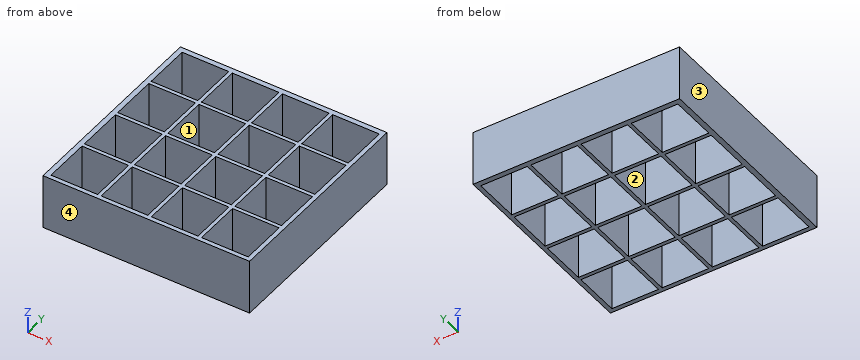
```python
from build123d import *

# Parameters (mm, degrees)
F0_W     = 1463.675
F0_H     = 1463.675
F0_W_2   = 330.2
F0_H_2   = 330.2
F1_DEPTH = 390.525
F2_SCALE = 0.05


with BuildPart() as f1:
    # F0 (on Top) → F1 (new body)
    with BuildSketch(Plane.XY):
        Rectangle(F0_W, F0_H)
        with Locations((-530.225, -536.575)):
            Rectangle(F0_W_2, F0_H_2, mode=Mode.SUBTRACT)
        with Locations((-174.625, -536.575)):
            Rectangle(F0_W_2, F0_H_2, mode=Mode.SUBTRACT)
        with Locations((-530.225, -180.975)):
            Rectangle(F0_W_2, F0_H_2, mode=Mode.SUBTRACT)
        with Locations((-174.625, -180.975)):
            Rectangle(F0_W_2, F0_H_2, mode=Mode.SUBTRACT)
        with Locations((180.975, -536.575)):
            Rectangle(F0_W_2, F0_H_2, mode=Mode.SUBTRACT)
        with Locations((536.575, -536.575)):
            Rectangle(F0_W_2, F0_H_2, mode=Mode.SUBTRACT)
        with Locations((180.975, -180.975)):
            Rectangle(F0_W_2, F0_H_2, mode=Mode.SUBTRACT)
        with Locations((536.575, -180.975)):
            Rectangle(F0_W_2, F0_H_2, mode=Mode.SUBTRACT)
        with Locations((-530.225, 174.625)):
            Rectangle(F0_W_2, F0_H_2, mode=Mode.SUBTRACT)
        with Locations((-174.625, 174.625)):
            Rectangle(F0_W_2, F0_H_2, mode=Mode.SUBTRACT)
        with Locations((-530.225, 530.225)):
            Rectangle(F0_W_2, F0_H_2, mode=Mode.SUBTRACT)
        with Locations((-174.625, 530.225)):
            Rectangle(F0_W_2, F0_H_2, mode=Mode.SUBTRACT)
        with Locations((180.975, 174.625)):
            Rectangle(F0_W_2, F0_H_2, mode=Mode.SUBTRACT)
        with Locations((536.575, 174.625)):
            Rectangle(F0_W_2, F0_H_2, mode=Mode.SUBTRACT)
        with Locations((180.975, 530.225)):
            Rectangle(F0_W_2, F0_H_2, mode=Mode.SUBTRACT)
        with Locations((536.575, 530.225)):
            Rectangle(F0_W_2, F0_H_2, mode=Mode.SUBTRACT)
    extrude(amount=F1_DEPTH)


with BuildPart() as f1_1:
    # F2: moved
    add(f1.part.scale(F2_SCALE))


solid = f1_1.part
```
Input: part model. Units: mm. Frame: model coordinates. Face numbers are marked on the shaded views. Coordinates: 2 decimals unless noted, no trailing zeros. Write each loop counter-clockwise with the first axis right and the second up, starting at its lowest first coordinate (ties: lowest second). Pieces come first, ordered by that corner, then holes. Notation, with made-up numbers: M 71,76 L 110,76 A20 cw 110,89 Z; hole C 85,-22.5 d2. An arc over 180 degrees is marked long. Use one line per item in the form item = value.
Q1. Section C-C (z = 1.5). Count the separate pieces of the cut face and the enclosed holes in it, plus the area to 3 significant figures.
Answer below:
separate_pieces = 1
enclosed_holes = 16
area = 995 mm²
Q2. Material intervals for probe 1 along X at (y, z) = (32, 10.5); probe 2 along Y at (x, z) = (-29, 17.25), sorted ascending. Write a range as from..to.
Answer below:
probe_1 = -36.59..-34.77, -18.26..-16.99, -0.48..0.79, 17.3..18.57, 35.08..36.59
probe_2 = -36.59..-35.08, -18.57..-17.3, -0.79..0.48, 16.99..18.26, 34.77..36.59
Q3. Draft query along Y for the marked faces 1, 2, 3 and 4. Return one class per face: released by +Y, released by -Y, zero draft, split by the parting line, or undercut.
Answer below:
face_1 = undercut
face_2 = undercut
face_3 = zero draft
face_4 = released by -Y
Q4. Section A-A (y = -8.5). Return loops of the section in (x, z), plus the area to 3 significant figures.
Answer below:
outline = M -36.59,0 L -34.77,0 L -34.77,19.53 L -36.59,19.53 Z; M -18.26,0 L -16.99,0 L -16.99,19.53 L -18.26,19.53 Z; M -0.48,0 L 0.79,0 L 0.79,19.53 L -0.48,19.53 Z; M 17.3,0 L 18.57,0 L 18.57,19.53 L 17.3,19.53 Z; M 35.08,0 L 36.59,0 L 36.59,19.53 L 35.08,19.53 Z
area = 139 mm²
Q5. Section B-B (x = -23.5). Return loops of the section in (y, z).
Answer below:
outline = M -36.59,0 L -35.08,0 L -35.08,19.53 L -36.59,19.53 Z; M -18.57,0 L -17.3,0 L -17.3,19.53 L -18.57,19.53 Z; M -0.79,0 L 0.48,0 L 0.48,19.53 L -0.79,19.53 Z; M 16.99,0 L 18.26,0 L 18.26,19.53 L 16.99,19.53 Z; M 34.77,0 L 36.59,0 L 36.59,19.53 L 34.77,19.53 Z
